The listing builds one solid part. Answer for the finished solid, in the listing's coordinates (mm). Face numbers are marked on the shaded views. A direction names the side the tool comes from. Coordinates: 2 decimals unless noted, no trailing zeros. Order: outer loops, then holes, each group sorted by start corner. A loop starts at its lowest first (then second) coordinate and runs counter-clockwise, first axis right, second up.
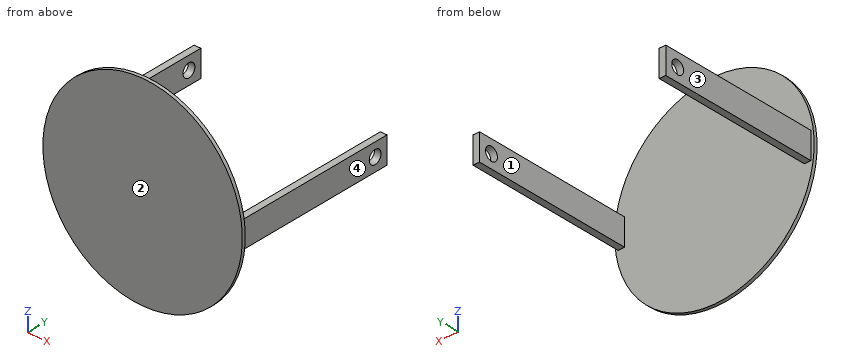
from build123d import *

# Parameters (mm, degrees)
SZKIC1_W                      = 10
SZKIC1_H                      = 40
DODANIE_WYCI_GNI_CIE1_DEPTH   = 250
DODANIE_WYCI_GNI_CIE1_2_DEPTH = 250
SZKIC1_3_R                    = 150
DODANIE_WYCI_GNI_CIE2_DEPTH   = 5
SZKIC2_R                      = 10
WYTNIJ_WYCI_GNI_CIE1_DEPTH    = 290


with BuildPart() as part:
    # Szkic1 → Dodanie-wyci_gni_cie1 (new body)
    with BuildSketch(Plane(origin=(0, 0, 0), x_dir=(1, 0, 0), z_dir=(0, 1, 0))):
        with Locations((140, 0)):
            Rectangle(SZKIC1_W, SZKIC1_H)
    extrude(amount=DODANIE_WYCI_GNI_CIE1_DEPTH)



with BuildPart() as body_2:
    # Szkic1 → Dodanie-wyci_gni_cie1 2 (new body)
    with BuildSketch(Plane(origin=(0, 0, 0), x_dir=(1, 0, 0), z_dir=(0, 1, 0))):
        with Locations((-140, 0)):
            Rectangle(SZKIC1_W, SZKIC1_H)
    extrude(amount=DODANIE_WYCI_GNI_CIE1_2_DEPTH)


with BuildPart() as part_1:
    add(part.part)

    add(body_2.part)  # Dodanie-wyci_gni_cie2 merges body 2
    # Szkic1_3 → Dodanie-wyci_gni_cie2 (add)
    with BuildSketch(Plane(origin=(0, 0, 0), x_dir=(1, 0, 0), z_dir=(0, 1, 0))):
        with Locations(Location((0, 0, 0), (0, 0, 270))):
            Circle(SZKIC1_3_R)
    extrude(amount=DODANIE_WYCI_GNI_CIE2_DEPTH)

    # Szkic2 → Wytnij-wyci_gni_cie1 (cut)
    with BuildSketch(Plane(origin=(145, 0, 0), x_dir=(0, 0, -1), z_dir=(1, 0, 0))):
        with Locations((0, 230)):
            Circle(SZKIC2_R)
    extrude(amount=-WYTNIJ_WYCI_GNI_CIE1_DEPTH, mode=Mode.SUBTRACT)


solid = part_1.part
1) Each of these flat-tipped pins is pushed along its axis until it touches: P1, Ø3, axis at x = 138.5, y = 87.5, coming from the +Z side; P2, Ø5, axis at x = 60.5, z = 52, coming from the +Y side; P3, Ø20, axis at y = 117, z = -0.5, coming from the -X side; P4, Ø18, axis at y = 230, z = 0, coming from the -X side. Where does it stop, or does it pass through?
2) A tool of negligible diameter and unlimited length cuts with its end or side. For the marked faces 1, 2, 3 and 4, from which of +Z, -Z, +X, -X, +Y, -Y can it reach the whole face along a straight path? Write none if from no direction.
3) Section C-C (y = 230) is taken. Give the vertices of the cut face in (x, z).
4) Section D-D (x = 0) is taken. Give the vertices of the cut face in (y, z).
5) Section A-A (y = 122.5) is taken. Give the vertices of the cut face in (x, z).
6) Consider L1, parallel to Y at x = 138.25, z = 0; L2, parallel to X at y = 210.5, z = -12; L3, parallel to Y at x = 71.5, z = -77. Determine where each line is inside the solid, lowest interval first.
7) Section B-B (z = 0) is taken. Give the vertices of the cut face in (x, y).
Filled sheet:
1. P1: stops at z = 20
1. P2: stops at y = 5
1. P3: stops at x = -145
1. P4: passes through
2. face 1: +Z, -Z, +Y
2. face 2: +Z, -Z, +X, -X, -Y
2. face 3: +Z, -Z, -X, +Y
2. face 4: +Z, -Z, +X, +Y
3. outline: (-145, -20) - (-135, -20) - (-135, -10) - (-145, -10) - close; (-145, 10) - (-135, 10) - (-135, 20) - (-145, 20) - close; (135, -20) - (145, -20) - (145, -10) - (135, -10) - close; (135, 10) - (145, 10) - (145, 20) - (135, 20) - close
4. outline: (0, -150) - (5, -150) - (5, 150) - (0, 150) - close
5. outline: (-145, -20) - (-135, -20) - (-135, 20) - (-145, 20) - close; (135, -20) - (145, -20) - (145, 20) - (135, 20) - close
6. L1: y = 0 to 220, 240 to 250
6. L2: x = -145 to -135, 135 to 145
6. L3: y = 0 to 5
7. outline: (-150, 0) - (150, 0) - (150, 5) - (145, 5) - (145, 220) - (135, 220) - (135, 5) - (-135, 5) - (-135, 220) - (-145, 220) - (-145, 5) - (-150, 5) - close; (-145, 240) - (-135, 240) - (-135, 250) - (-145, 250) - close; (135, 240) - (145, 240) - (145, 250) - (135, 250) - close
